```python
from build123d import *

# Parameters (mm, degrees)
SKETCH1_W           = 138.1
SKETCH1_H           = 57.1
SKETCH1_R           = 2.5
SKETCH1_R_2         = 11
BOSS_EXTRUDE1_DEPTH = 4.7625


with BuildPart() as part:
    # Sketch1 → Boss-Extrude1 (new body)
    with BuildSketch(Plane.ZY.offset(82.970238089)):
        with Locations((-89.208048627, -51.057798632)):
            Rectangle(SKETCH1_W, SKETCH1_H)
        with Locations(Location((-153.258048627, -27.507798632, 0), (0, 0, 90))):
            Circle(SKETCH1_R, mode=Mode.SUBTRACT)
        with Locations(Location((-153.258048627, -74.607798632, 0), (0, 0, 90))):
            Circle(SKETCH1_R, mode=Mode.SUBTRACT)
        with Locations(Location((-25.158048627, -27.507798632, 0), (0, 0, 90))):
            Circle(SKETCH1_R, mode=Mode.SUBTRACT)
        with Locations(Location((-25.158048627, -74.607798632, 0), (0, 0, 90))):
            Circle(SKETCH1_R, mode=Mode.SUBTRACT)
        with Locations(Location((-48.708048627, -51.057798632, 0), (0, 0, 90))):
            Circle(SKETCH1_R_2, mode=Mode.SUBTRACT)
    extrude(amount=BOSS_EXTRUDE1_DEPTH)


solid = part.part
```
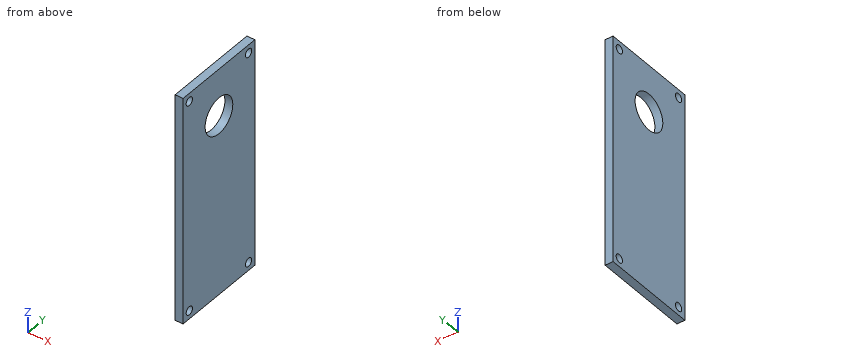
Model file for the job. Use its own axes, mm. Coordinates: 2 decimals unless noted, no trailing zeros. Write each loop counter-clockwise with the first axis right and the second up, starting at its lowest first coordinate (ties: lowest second). Pieces come first, ordered by that corner, then holes. Notation, with made-up numbers: (32.25, 82.25) - (78.25, 82.25) arc R11 ccw to (78.25, 97.25) - close; hole circle Ø8 at (75.5, 28). An arc over 180 degrees is marked (long way). One line per item, written item: value. Start each with the question number.
1. Slice it at A-A (y = -74). Write the cut outline in (x, z), plus the area to 3 significant figures.
2. Slice it at C-C (y = -42). Write the cut outline in (x, z), plus the area to 3 significant figures.
3. Flat gauge pin, fed straight in: pin 1 (13 mm diameter, centred on y = -51.06, z = -48.71, fed in from -X). Where does the tip first touch, or does it go through?
4. Slice it at D-D (z = -45.5). Write the cut outline in (x, y).
5. Probe line 1 (Z direction, x = -86.8, y = -26); line 2 (Z direction, x = -85.4, y = -42.5); line 3 (Y direction, x = -83.85, z = -58.5). List the from-to ranges inside material, lowest first. Write a range as from..to.
6. Slice it at B-B (x = -85). Write the cut outline in (y, z).
Answers below:
1. outline: (-87.73, -158.26) - (-82.97, -158.26) - (-82.97, -155.68) - (-87.73, -155.68) - close; (-87.73, -150.83) - (-82.97, -150.83) - (-82.97, -27.58) - (-87.73, -27.58) - close; (-87.73, -22.73) - (-82.97, -22.73) - (-82.97, -20.16) - (-87.73, -20.16) - close
1. area: 612 mm^2
2. outline: (-87.73, -158.26) - (-82.97, -158.26) - (-82.97, -54.95) - (-87.73, -54.95) - close; (-87.73, -42.47) - (-82.97, -42.47) - (-82.97, -20.16) - (-87.73, -20.16) - close
2. area: 598 mm^2
3. pin 1: passes through
4. outline: (-87.73, -79.61) - (-82.97, -79.61) - (-82.97, -61.58) - (-87.73, -61.58) - close; (-87.73, -40.54) - (-82.97, -40.54) - (-82.97, -22.51) - (-87.73, -22.51) - close
5. line 1: z = -158.26..-155.25, -151.26..-27.15, -23.16..-20.16
5. line 2: z = -158.26..-55.62, -41.8..-20.16
5. line 3: y = -79.61..-56.07, -46.05..-22.51
6. outline: (-79.61, -158.26) - (-22.51, -158.26) - (-22.51, -20.16) - (-79.61, -20.16) - close; hole circle Ø5 at (-74.61, -153.26); hole circle Ø5 at (-74.61, -25.16); hole circle Ø22 at (-51.06, -48.71); hole circle Ø5 at (-27.51, -153.26); hole circle Ø5 at (-27.51, -25.16)
